Build history of the part. All positions in model axes, mm. A direction names the side the tool comes from. Give positions to 0.01 mm unless a question says otherwise; leave off trailing zeros. Write each loop counter-clockwise with the first axis right and the second up, starting at its lowest first coordinate (ties: lowest second). Pieces come first, ordered by that corner, then holes. Notation, with made-up numbers: (-10.5, 0.25) - (28.5, 0.25) arc R15 cw to (28.5, 4.25) - close; hole circle Ø5 at (6, 89). An arc over 180 degrees is marked (long way). Use one line per item in the form item = value. Start each with the question number.
from build123d import *

# Parameters (mm, degrees)
CUT_EXTRUDE_1_DEPTH      = 10
CUT_EXTRUDE_1_DEPTH_BACK = 10
SKETCH_2_R               = 10


with BuildPart() as part:
    # Sketch 1 → Revolve 1 (revolve)
    with BuildSketch(Plane.XY, mode=Mode.PRIVATE) as revolve_1_sk:
        Polygon((-30, 50), (0, 50), (0, 0), (-35, 0), (-35, 300), (0, 300), (0, 280), (-30, 280), align=None)
    revolve(revolve_1_sk.sketch.rotate(Axis((0, 50, 0), (0, -1, 0)), 270), axis=Axis((0, 50, 0), (0, -1, 0)))

    # Sketch 2 → Cut-Extrude 1 (cut, two sides: drawn at the far end of the back side and taken through both)
    with BuildSketch(Plane.XY.offset(-32).offset(-CUT_EXTRUDE_1_DEPTH_BACK)):
        with Locations(Location((0, 25, 0), (0, 0, 180))):
            Circle(SKETCH_2_R)
    extrude(amount=CUT_EXTRUDE_1_DEPTH + CUT_EXTRUDE_1_DEPTH_BACK, mode=Mode.SUBTRACT)


solid = part.part
(1) Pin check, flat tips, straight feed: pin 1 Ø10 at (y, z) = (107, 1) entering from -X; pin 2 Ø5 at (x, y) = (1.5, 31.5) entering from -Z; pin 3 Ø12 at (y, z) = (256, -17.5) entering from -X. Stop position of each tip, or through.
(2) Which spindle directions (+Z, -Z, +X, -X, +Y, -Y) get a long thin tool onto all of the face, cutting with end or side? Do faces 1 (the flat face through (0, 300, 0)), 2 (the cylindrical face through (-9.54, 22, -28.59)), 3 (the flat face through (0, 280, 0)). Say none if no direction does.
(3) Wall check: line 1 (Y direction, x = -3, z = -8.5); line 2 (X direction, y = 206, z = 0); line 3 (Y direction, x = 0, z = -24.75). Give the ranges that are in metal, low to high. Write a range as from..to.
(4) Cut at B-B, the plane z = 0. Give the cut face in (x, y).
(5) Cut at A-A, the plane x = 0. Give the cut face in (y, z), then the cut area to 3 significant figures.
(6) Cut at C-C, the plane y = 109. Give the cut face in (x, z), then the cut area to 3 significant figures.
(7) Cut at D-D, the plane z = 20.5. Give the cut face in (x, y), then the cut area to 3 significant figures.
(8) Two-plate mould, pull along X, no slides. Class faces 4 (the flat face through (0, 50, 0)), 5 (the flat face through (0, 0, 0)), 6 (the cylindrical face through (-10.513, 152.1, 33.384)): +X half, -X half, draft (parallel to the pull), parting line (faces both ways), or undercut.
Solution:
q1.pin_1 = -35
q1.pin_2 = -22
q1.pin_3 = -33.06
q2.face_1 = +Z, -Z, +X, -X, +Y
q2.face_2 = -Z
q2.face_3 = none
q3.line_1 = 0..50, 280..300
q3.line_2 = -35..-30, 30..35
q3.line_3 = 0..15, 35..50, 280..300
q4.outline = (-35, 0) - (35, 0) - (35, 300) - (-35, 300) - close; hole (-30, 50) - (30, 50) - (30, 280) - (-30, 280) - close
q5.outline = (0, -35) - (15, -35) - (15, -22) - (35, -22) - (35, -35) - (300, -35) - (300, 35) - (0, 35) - close; hole (50, -30) - (280, -30) - (280, 30) - (50, 30) - close
q5.area = 6,940 mm2
q6.outline = circle Ø70 at (0, 0); hole circle Ø60 at (0, 0)
q6.area = 1,020 mm2
q7.outline = (-28.37, 0) - (28.37, 0) - (28.37, 300) - (-28.37, 300) - close; hole (-21.9, 50) - (21.9, 50) - (21.9, 280) - (-21.9, 280) - close
q7.area = 6,950 mm2
q8.face_4 = undercut
q8.face_5 = draft
q8.face_6 = parting line
